Design review of the part built by this model. Coordinates are the model's own, in mm. Face numbers are marked on the shaded views. A direction names the side the tool comes from. Give positions to 0.01 mm unless a question says otherwise; leave off trailing zeros. Order: outer loops, then holes, each group sorted by start corner. A loop starts at its lowest first (then second) coordinate and runs counter-clockwise, first axis right, second up. Notation, with made-up numbers: M 25.5,21.5 L 39.5,21.5 A23 ccw 39.5,57.5 Z; hole C -19.75,44 d9. An arc over 180 degrees is marked long. Answer as a JSON object with one key per item and string values.
from build123d import *

# Parameters (mm, degrees)
SKETCH1_W                = 90
SKETCH1_H                = 90
BOSS_EXTRUDE1_DEPTH      = 3
BOSS_EXTRUDE3_DEPTH      = 2.5
SKETCH6_W                = 90
SKETCH6_H                = 90
SKETCH6_W_2              = 88
SKETCH6_H_2              = 88
BOSS_EXTRUDE4_DEPTH      = 15
BOSS_EXTRUDE4_DEPTH_BACK = 10


with BuildPart() as part:
    # Sketch1 → Boss-Extrude1 (new body)
    with BuildSketch(Plane(origin=(0, 0, 0), x_dir=(1, 0, 0), z_dir=(0, 1, 0))):
        Rectangle(SKETCH1_W, SKETCH1_H)
    extrude(amount=BOSS_EXTRUDE1_DEPTH)

    # Sketch4 → Boss-Extrude3 (add)
    with BuildSketch(Plane(origin=(0, 3, 0), x_dir=(1, 0, 0), z_dir=(0, 1, 0))):
        Polygon((6.366838491, 0.875), (6.366838491, -0.875), (7.983419247, -3.675000002), (11.216580757, -3.675000001), (12.833161509, -0.875), (12.833161509, 0), (12.833161509, 0.875), (11.216580757, 3.675000001), (7.983419247, 3.675000002), align=None)
        Polygon((6.366838491, 19.475), (6.366838491, 17.725), (7.983419247, 14.924999998), (11.216580757, 14.924999999), (12.833161509, 17.725), (12.833161509, 18.6), (12.833161509, 19.475), (11.216580757, 22.275000001), (7.983419247, 22.275000002), align=None)
        Polygon((24.966838491, 0.875), (24.966838491, -0.875), (26.583419247, -3.675000002), (29.816580757, -3.675000001), (31.433161509, -0.875), (31.433161509, 0), (31.433161509, 0.875), (29.816580757, 3.675000001), (26.583419247, 3.675000002), align=None)
        Polygon((24.966838491, -17.725), (24.966838491, -19.475), (26.583419247, -22.275000002), (29.816580757, -22.275000001), (31.433161509, -19.475), (31.433161509, -18.6), (31.433161509, -17.725), (29.816580757, -14.924999999), (26.583419247, -14.924999998), align=None)
        Polygon((6.366838491, -17.725), (6.366838491, -19.475), (7.983419247, -22.275000002), (11.216580757, -22.275000001), (12.833161509, -19.475), (12.833161509, -18.6), (12.833161509, -17.725), (11.216580757, -14.924999999), (7.983419247, -14.924999998), align=None)
        Polygon((-30.833161509, 0.875), (-30.833161509, -0.875), (-29.216580753, -3.675000002), (-25.983419243, -3.675000001), (-24.366838491, -0.875), (-24.366838491, 0), (-24.366838491, 0.875), (-25.983419243, 3.675000001), (-29.216580753, 3.675000002), align=None)
        Polygon((-12.233161509, 0.875), (-12.233161509, -0.875), (-10.616580753, -3.675000002), (-7.383419243, -3.675000001), (-5.766838491, -0.875), (-5.766838491, 0), (-5.766838491, 0.875), (-7.383419243, 3.675000001), (-10.616580753, 3.675000002), align=None)
        Polygon((-12.233161509, -17.725), (-12.233161509, -19.475), (-10.616580753, -22.275000002), (-7.383419243, -22.275000001), (-5.766838491, -19.475), (-5.766838491, -18.6), (-5.766838491, -17.725), (-7.383419243, -14.924999999), (-10.616580753, -14.924999998), align=None)
        Polygon((-30.833161509, -17.725), (-30.833161509, -19.475), (-29.216580753, -22.275000002), (-25.983419243, -22.275000001), (-24.366838491, -19.475), (-24.366838491, -18.6), (-24.366838491, -17.725), (-25.983419243, -14.924999999), (-29.216580753, -14.924999998), align=None)
        Polygon((24.966838491, 19.475), (24.966838491, 17.725), (26.583419247, 14.924999998), (29.816580757, 14.924999999), (31.433161509, 17.725), (31.433161509, 18.6), (31.433161509, 19.475), (29.816580757, 22.275000001), (26.583419247, 22.275000002), align=None)
        Polygon((-30.833161509, 19.475), (-30.833161509, 17.725), (-29.216580753, 14.924999998), (-25.983419243, 14.924999999), (-24.366838491, 17.725), (-24.366838491, 18.6), (-24.366838491, 19.475), (-25.983419243, 22.275000001), (-29.216580753, 22.275000002), align=None)
        Polygon((-12.233161509, 19.475), (-12.233161509, 17.725), (-10.616580753, 14.924999998), (-7.383419243, 14.924999999), (-5.766838491, 17.725), (-5.766838491, 18.6), (-5.766838491, 19.475), (-7.383419243, 22.275000001), (-10.616580753, 22.275000002), align=None)
    extrude(amount=BOSS_EXTRUDE3_DEPTH)

    # Sketch6 → Boss-Extrude4 (add, two sides)
    with BuildSketch(Plane(origin=(0, 3, 0), x_dir=(1, 0, 0), z_dir=(0, 1, 0))) as boss_extrude4_sk:
        Rectangle(SKETCH6_W, SKETCH6_H)
        Rectangle(SKETCH6_W_2, SKETCH6_H_2, mode=Mode.SUBTRACT)
    extrude(amount=BOSS_EXTRUDE4_DEPTH)
    extrude(boss_extrude4_sk.sketch, amount=-BOSS_EXTRUDE4_DEPTH_BACK)


solid = part.part
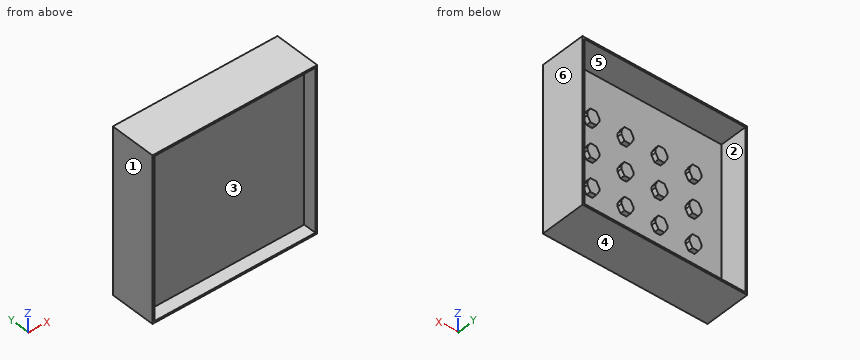
(1) We need section C-C (z = 5.5). Write out the cut boundary in (x, y), plus the area to 3 significant figures.
Checked values:
{"outline": "M -45,-7 L -44,-7 L -44,0 L 44,0 L 44,-7 L 45,-7 L 45,18 L 44,18 L 44,3 L -44,3 L -44,18 L -45,18 Z", "area": "314 mm^2"}
(2) We need section A-A (y = 13.25). Write out the cut boundary in (x, z).
Checked values:
{"outline": "M -45,-45 L 45,-45 L 45,45 L -45,45 Z; hole M -44,-44 L 44,-44 L 44,44 L -44,44 Z"}
(3) Tool access review of the marked faces 1, 2 and 3: name each direction out of +Z, -Z, +X, -X, +Y, -Y from which nothing blocks a thin tool from reaching the whole face with its end or side.
Checked values:
{"face 1": "+Z, -Z, -X, +Y, -Y", "face 2": "+Y", "face 3": "-Y"}
(4) We need section D-D (z = 16.5). Write out the cut boundary in (x, y).
Checked values:
{"outline": "M -45,-7 L -44,-7 L -44,0 L 44,0 L 44,-7 L 45,-7 L 45,18 L 44,18 L 44,3 L 30.73,3 L 30.73,5.5 L 25.67,5.5 L 25.67,3 L 12.13,3 L 12.13,5.5 L 7.07,5.5 L 7.07,3 L -6.47,3 L -6.47,5.5 L -11.53,5.5 L -11.53,3 L -25.07,3 L -25.07,5.5 L -30.13,5.5 L -30.13,3 L -44,3 L -44,18 L -45,18 Z"}
(5) To check wall thickness, follow L1, parallel to X at y = -4.75, z = 6; L2, parallel to Z at x = -11, y = 3.25. State the ranges of each line that lie inside material, in increasing order. Write a range as from..to.
Checked values:
{"L1": "x = -45..-44, 44..45", "L2": "z = -45..-44, -21.61..-15.59, -3.01..3.01, 15.59..21.61, 44..45"}
(6) Insertion check: pin 1 (10 mm diameter, centred on x = 23.5, z = -15, fed in from +Y); pin 2 (1.5 mm diameter, centred on x = -32, z = -16.5, fed in from -Y). Each pin has a flat end and moves straight along its axis. Give the tip position at first contact, or say it passes through.
Checked values:
{"pin 1": "stops at y = 5.5", "pin 2": "stops at y = 0"}
(7) We need section B-B (x = 1.5). Write out the cut boundary in (y, z).
Checked values:
{"outline": "M -7,-45 L 18,-45 L 18,-44 L 3,-44 L 3,44 L 18,44 L 18,45 L -7,45 L -7,44 L 0,44 L 0,-44 L -7,-44 Z"}
(8) Draft analysis for pull direction X (two halves, no side actions). For the marked faces 4, 5 and 6, state which applies: +X half, -X half, draft (parallel to the pull), parting line (faces both ways), or undercut.
Checked values:
{"face 4": "draft", "face 5": "undercut", "face 6": "+X half"}
